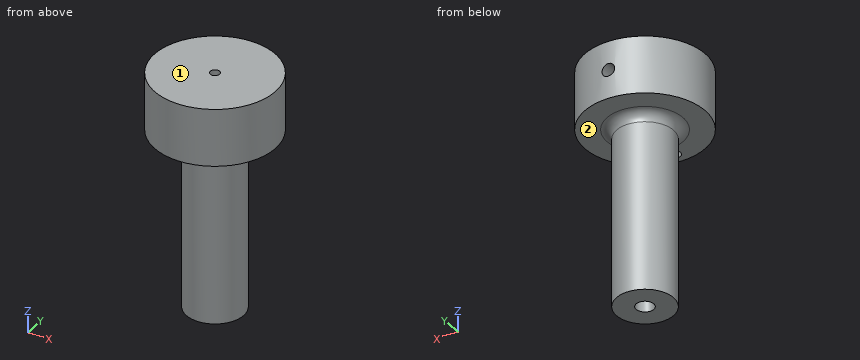
from build123d import *

# Parameters (mm, degrees)
SZKIC2_W = 56
SZKIC2_H = 9
SZKIC3_W = 18
SZKIC3_H = 19


with BuildPart() as part:
    # Szkic2 → Obr_t1 (revolve)
    with BuildSketch(Plane(origin=(0, 0, 0), x_dir=(0, 0, -1), z_dir=(1, 0, 0)), mode=Mode.PRIVATE) as obr_t1_sk:
        with Locations((-28, 4.5)):
            Rectangle(SZKIC2_W, SZKIC2_H)
    revolve(obr_t1_sk.sketch.rotate(Axis((0, 0, 0), (0, 0, 1)), 270), axis=Axis((0, 0, 0), (0, 0, 1)))

    # Szkic3 → Obr_t2 (revolve)
    with BuildSketch(Plane(origin=(0, 0, 0), x_dir=(0, 0, -1), z_dir=(1, 0, 0)), mode=Mode.PRIVATE) as obr_t2_sk:
        with Locations((-65, 9.5)):
            Rectangle(SZKIC3_W, SZKIC3_H)
    revolve(obr_t2_sk.sketch.rotate(Axis((0, 0, 56), (0, 0, 1)), 270), axis=Axis((0, 0, 56), (0, 0, 1)))

    # Szkic4 → Wyci_cie-obr_t1 (revolve, cut)
    with BuildSketch(Plane(origin=(0, 0, 0), x_dir=(0, 0, -1), z_dir=(1, 0, 0)), mode=Mode.PRIVATE) as wyci_cie_obr_t1_sk:
        Polygon((-74, 0), (-74, 1.5), (0, 2.791674805), (0, 0), align=None)
    revolve(wyci_cie_obr_t1_sk.sketch.rotate(Axis((0, 0, 0), (0, 0, 1)), 270), axis=Axis((0, 0, 0), (0, 0, 1)), mode=Mode.SUBTRACT)

    # Szkic5 → Wyci_cie-obr_t2 (revolve, cut)
    with BuildSketch(Plane(origin=(0, 0, 0), x_dir=(0, 0, -1), z_dir=(1, 0, 0)), mode=Mode.PRIVATE) as wyci_cie_obr_t2_sk:
        Polygon((-65, 11.845299462), (-67, 13), (-67, 19), (-65, 19), align=None)
    revolve(wyci_cie_obr_t2_sk.sketch.rotate(Axis((0, 19, 65), (0, -1, 0)), 180), axis=Axis((0, 19, 65), (0, -1, 0)), mode=Mode.SUBTRACT)

    # Szkic6 → Obr_t3 (revolve)
    with BuildSketch(Plane(origin=(0, 0, 0), x_dir=(0, 0, -1), z_dir=(1, 0, 0)), mode=Mode.PRIVATE) as obr_t3_sk:
        with BuildLine():
            Line((-56, 9), (-53, 9))
            ThreePointArc((-53, 9), (-55.121320344, 9.878679656), (-56, 12))
            Line((-56, 12), (-56, 9))
        make_face()
    revolve(obr_t3_sk.sketch.rotate(Axis((0, 0, 0), (0, 0, 1)), 270), axis=Axis((0, 0, 0), (0, 0, 1)))

    # Szkic1 → Wyci_cie-obr_t3 (revolve, cut)
    with BuildSketch(Plane(origin=(0, -15, 0), x_dir=(1, 0, 0), z_dir=(0, 1, 0)), mode=Mode.PRIVATE) as wyci_cie_obr_t3_sk:
        Polygon((0, -56), (2, -56), (2, -62), (0, -63.154700538), align=None)
    revolve(wyci_cie_obr_t3_sk.sketch.rotate(Axis((0, -15, 63.154700538), (0, 0, -1)), 180), axis=Axis((0, -15, 63.154700538), (0, 0, -1)), mode=Mode.SUBTRACT)


solid = part.part
Could you check a few things on this model? Use its own coordinates, in mm. Face numbers are marked on the shaded views. A direction names the side the tool comes from. Give positions to 0.01 mm unless a question says otherwise; leave off trailing zeros. Order: outer loops, then holes, each group sorted by start corner. A loop starts at its lowest first (then second) coordinate and runs counter-clockwise, first axis right, second up. Notation, with made-up numbers: (-20.5, 36) - (20.5, 36) arc R19 ccw to (20.5, 71) - close; hole circle Ø11 at (82, 87). An arc over 180 degrees is marked (long way). Return JSON: item names as keys, results as strings. Group by question number.
Q1. Which directions (+Z, -Z, +X, -X, +Y, -Y) give clear straight access to the entire face, cutting with the end or side of a thin tool? Please do the marked faces 1 and 2.
Q2. Will these pins go through, and if not, where does the flat tip stop? pin 1 Ø12 at (x, y) = (12, -11.5) entering from -Z; pin 2 Ø4 at (y, z) = (0.5, 40) entering from -X; pin 3 Ø6 at (y, z) = (-2, 63.5) entering from +X; pin 4 Ø2 at (x, z) = (-0.5, 43) entering from -Y.
Q3. Please list where these lines run through material, in increasing order: line 1 along Z through (x, y) = (0, 16.5); line 2 along Z through (x, y) = (13, 10.5); line 3 along X through (y, z) = (14.5, 65). Write a range as [from, to].
Q4. Suppose I cut it at A-A, the plane z = 50. Please give me the cut outline in (x, y).
Q5. Suppose I cut it at B-B, the plane z = 8. Please give me the cut outline in (x, y).
Resolved:
{
 "1": {"face 1": "+Z, +X, -X, +Y, -Y", "face 2": "-Z"},
 "2": {"pin 1": "stops at z = 55.66", "pin 2": "stops at x = -9", "pin 3": "stops at x = 19", "pin 4": "stops at y = -9"},
 "3": {"line 1": "z = [56, 63], [67, 74]", "line 2": "z = [56, 74]", "line 3": "x = [-12.28, -2], [2, 12.28]"},
 "4": {"outline": "circle Ø18 at (0, 0); hole circle Ø3.84 at (0, 0)"},
 "5": {"outline": "circle Ø18 at (0, 0); hole circle Ø5.3 at (0, 0)"}
}
